from build123d import *

# Parameters (mm, degrees)
F3_W   = 53.975
F3_H   = 9.525
F3_W_2 = 9.525
F3_H_2 = 53.975


with BuildPart() as f4:
    # F4: sweep along a path in F1, F0, F1
    with BuildLine(Plane.XY) as f4_path:
        Line((0, 0), (0, -428.9635121822))
    with BuildLine(Plane.XZ) as f4_path_2:
        Line((0, 0), (200.792491436, 260.2265179157))
        Line((200.792491436, 260.2265179157), (475.3324985504, 260.2265179157))
        Line((475.3324985504, 260.2265179157), (749.8725056648, 260.2265179157))
        Line((749.8725056648, 260.2265179157), (950.6649971008, 0))
    with BuildLine(Plane.XY) as f4_path_3:
        Line((950.6649971008, 0), (950.6649971008, -428.9635121822))
    # F3 (on plane+point) → F4 (sweep)
    with BuildSketch(Plane.XZ.offset(428.9635121822)):
        with Locations((-26.9875, 4.7625)):
            Rectangle(F3_W, F3_H)
        with Locations((-58.7375, 36.5125)):
            Rectangle(F3_W_2, F3_H_2)
        with Locations((-58.7375, 4.7625)):
            Rectangle(F3_W_2, F3_H)
    sweep(path=f4_path.line + f4_path_2.line + f4_path_3.line, transition=Transition.RIGHT)


solid = f4.part
Work out the finished part from the listing and answer in its coordinate system (mm). A direction names the side the tool comes from. Coordinates: 2 decimals unless noted, no trailing zeros. Write each loop counter-clockwise with the first axis right and the second up, starting at its lowest first coordinate (ties: lowest second). Pieces come first, ordered by that corner, then holes. Notation, with made-up numbers: M 32.5,58.5 L 71.5,58.5 A25 cw 71.5,80.5 Z; hole C 32,14.25 d6. An arc over 180 degrees is marked long. Use one line per item in the form item = value. Start each with the question number.
1. A tool of negligible diameter and unlimited length cuts with its end or side. For faces 4 (the face through (74.24, 19.67, 137.94)), 5 (the face through (-32, -198, 0)), 6 (the face through (77.014, 8.715, 143.821)), from which of +Z, -Z, +X, -X, +Y, -Y can it reach the whole face along a straight path? Write none if from no direction.
2. The part is cut by section C-C (x = 666.5). Give the vertices of the cut face in (y, z).
3. The mould has two halves that part along Z. Classify faces 1 (the face through (471.155, 8.715, 287.113)), 2 (the face through (97.58, -3.72, 131.16)), 3 (the face through (-63.5, -198, 32)): released by +Z, released by -Z, zero draft, split by the parting line, or undercut.
4. The part is cut by section B-B (z = 192.5). Give the vertices of the cut face in (x, y).
5. The part is cut by section A-A (y = -37.5). Give the vertices of the cut face in (x, z) (3 decimals).
6. The part is cut by section D-D (z = 51). Give the vertices of the cut face in (x, y) (3 decimals), plus the area to 3 significant figures.
7. Straight lines are drawn through the part: probe 1 along X at (y, z) = (-7, 24) (3 decimals); probe 2 along Y at (x, z) = (380, 271); probe 3 along Y at (x, z) = (80, 247.5). For each, find the intervals that lie inside material, in ascending order. Write a range as from..to.
8. Each of these flat-tipped pins is pushed along its axis until it touches: P1, Ø8, axis at x = 585.5, y = -24, coming from the +Z side; P2, Ø5, axis at x = -59.5, y = -180.5, coming from the +Z side; P3, Ø3, axis at x = 64, z = 179, coming from the -Y side; P4, Ø8, axis at x = 298, z = 284, coming from the +Y side. Where does it stop, or does it pass through?
Evaluation:
q1.face_4 = -Z, +Y
q1.face_5 = -Z, +X, -X, +Y, -Y
q1.face_6 = -Y
q2.outline = M -17.3,341.75 L 25.43,308.78 L -7.54,266.05 L 0,260.23 L 38.79,310.5 L -11.48,349.29 Z
q3.face_1 = undercut
q3.face_2 = released by -Z
q3.face_3 = zero draft
q4.outline = M 36.04,-11.48 L 45.56,-17.3 L 87.21,25.43 L 141.18,-7.54 L 148.53,0 L 85.03,38.79 Z; M 802.13,0 L 809.48,-7.54 L 863.46,25.43 L 905.1,-17.3 L 914.63,-11.48 L 865.63,38.79 Z
q5.outline = M -63.5,0 L 0,0 L 0,9.525 L -53.975,9.525 L -53.975,63.5 L -63.5,63.5 Z; M 950.665,0 L 1014.165,0 L 1014.165,63.5 L 1004.64,63.5 L 1004.64,9.525 L 950.665,9.525 Z
q6.outline = M -63.5,-428.964 L -53.975,-428.964 L -53.975,-7.405 L -21.973,25.432 L 32.002,-7.541 L 39.352,0 L -24.148,38.792 L -63.5,-1.586 Z; M 911.313,0 L 918.663,-7.541 L 972.638,25.432 L 1004.64,-7.405 L 1004.64,-428.964 L 1014.165,-428.964 L 1014.165,-1.586 L 974.813,38.792 Z
q6.area = 10,600 mm^2
q7.probe_1 = -63.5..-53.975, 10.283..11.696, 938.969..940.382, 1004.64..1014.165
q7.probe_2 = -3.72..8.31
q7.probe_3 = -12.41..-9.92
q8.P1 = through
q8.P2 = 63.5
q8.P3 = 10.36
q8.P4 = 21.43
